```python
from build123d import *

# Parameters (mm, degrees)
BOSS_EXTRUDE1_DEPTH      = 4.826
BOSS_EXTRUDE1_DEPTH_BACK = 0.666205528
SKETCH1_W                = 82.55
SKETCH1_H                = 82.55
SKETCH1_R                = 4.826
SKETCH1_R_2              = 7.9375
CHAMFER1_SIZE            = 9.652


with BuildPart() as part:
    # Sketch1 → Boss-Extrude1 (new, two sides: drawn at the far end of the back side and taken through both)
    with BuildSketch(Plane(origin=(106.639199962, 25.37693728, 0), x_dir=(1, 0, 0), z_dir=(0, 0, 1)).offset(-BOSS_EXTRUDE1_DEPTH_BACK)):
        with Locations((0, 320.675)):
            Rectangle(SKETCH1_W, SKETCH1_H)
        with Locations((-28.575, 347.6625)):
            Circle(SKETCH1_R, mode=Mode.SUBTRACT)
        with Locations((-28.575, 293.6875)):
            Circle(SKETCH1_R, mode=Mode.SUBTRACT)
        with Locations((28.575, 347.6625)):
            Circle(SKETCH1_R, mode=Mode.SUBTRACT)
        with Locations((28.575, 293.6875)):
            Circle(SKETCH1_R, mode=Mode.SUBTRACT)
        with Locations((0, 320.675)):
            Circle(SKETCH1_R_2, mode=Mode.SUBTRACT)
    extrude(amount=BOSS_EXTRUDE1_DEPTH + BOSS_EXTRUDE1_DEPTH_BACK)

    # Chamfer1
    chamfer1_edges = [part.edges().sort_by_distance(p)[0] for p in [
        (147.914199962, 304.77693728, 2.079897236),
        (65.364199962, 304.77693728, 2.079897236),
        (65.364199962, 387.32693728, 2.079897236),
        (147.914199962, 387.32693728, 2.079897236),
    ]]
    chamfer(chamfer1_edges, length=CHAMFER1_SIZE)


solid = part.part
```
Check sheet for the modelled part. Datum: model origin and axes. Units: mm. Coordinates: 2 decimals unless noted, no trailing zeros. Order: outer loops, then holes, each group sorted by start corner. A loop starts at its lowest first (then second) coordinate and runs counter-clockwise, first axis right, second up. Notation, with made-up numbers: (33.5, 73) -> (81.5, 73) arc R31 ccw to (81.5, 100) -> close; hole circle Ø1 at (89, 68.25). An arc over 180 degrees is marked (long way). Write item = value, one per line. Start each with the question number.
1) Go/stop test with a flat-tipped pin: P1, Ø6, axis at x = 135.21, y = 373.04, coming from the -Z side. Record where the tip stops, or that it passes through.
2) Mould release check, pull along X, two halves, no side actions. Record for faces 1 (the flat face through (143.156, 309.671, 2.041)), 2 (the flat face through (65.364, 346, 2)), 3 (the cylindrical face through (77.018, 368.328, 2.041)): +X half, -X half, draft (parallel to the pull), parting line (faces both ways), or undercut.
3) Cross-section at D-D (x = 81.5). Enter the section's corners in (y, z), then the cut area to 3 significant figures.
4) Cross-section at B-B (x = 106.5). Enter the section's corners in (y, z), then the cut area to 3 significant figures.
5) Material ranges on L1, parallel to Y at x = 107, z = 1.95; L2, parallel to Y at x = 132, z = 0.75; L3, parallel to Y at x = 136, z = 3.1, recorded low to high.
6) Cross-section at A-A (y = 371.5). Enter the section's corners in (x, z), then the cut area to 3 significant figures.
7) Cross-section at C-C (y = 351). Enter the section's corners in (x, z), then the cut area to 3 significant figures.
Ans:
q1.P1 = through
q2.face_1 = +X half
q2.face_2 = -X half
q2.face_3 = undercut
q3.outline = (304.78, -0.67) -> (315.68, -0.67) -> (315.68, 4.83) -> (304.78, 4.83) -> close; (322.45, -0.67) -> (369.65, -0.67) -> (369.65, 4.83) -> (322.45, 4.83) -> close; (376.43, -0.67) -> (387.33, -0.67) -> (387.33, 4.83) -> (376.43, 4.83) -> close
q3.area = 379 mm²
q4.outline = (304.78, -0.67) -> (338.12, -0.67) -> (338.12, 4.83) -> (304.78, 4.83) -> close; (353.99, -0.67) -> (387.33, -0.67) -> (387.33, 4.83) -> (353.99, 4.83) -> close
q4.area = 366 mm²
q5.L1 = 304.78 to 338.12, 353.98 to 387.33
q5.L2 = 304.78 to 315.46, 322.66 to 369.44, 376.64 to 387.33
q5.L3 = 304.78 to 314.3, 323.83 to 368.28, 377.8 to 387.33
q6.outline = (65.36, -0.67) -> (73.49, -0.67) -> (73.49, 4.83) -> (65.36, 4.83) -> close; (82.64, -0.67) -> (130.64, -0.67) -> (130.64, 4.83) -> (82.64, 4.83) -> close; (139.79, -0.67) -> (147.91, -0.67) -> (147.91, 4.83) -> (139.79, 4.83) -> close
q6.area = 353 mm²
q7.outline = (65.36, -0.67) -> (100.43, -0.67) -> (100.43, 4.83) -> (65.36, 4.83) -> close; (112.85, -0.67) -> (147.91, -0.67) -> (147.91, 4.83) -> (112.85, 4.83) -> close
q7.area = 385 mm²
